For this review, take the finished solid that the model builds, in its own axes (mm). A direction names the side the tool comes from. Round coordinates to 2 decimals unless told otherwise and drop trailing zeros. Loops run counter-clockwise (first coordinate to the right, second up) from the corner with the lowest first, then second, coordinate; pieces in that order, holes last. Notation, with made-up numbers: M 31.5,-8 L 90.5,-8 A30 ccw 90.5,16 Z; hole C 62,82.25 d7. An arc over 180 degrees is marked long. Write item = value, one per line. Start each with the question number.
Autodesk Inventor part; units mm, degrees
ref_plane "YZ Plane" through (0, 0, 0) normal (1, 0, 0) x (0, 1, 0)
ref_plane "XZ Plane" through (0, 0, 0) normal (0, 1, 0) x (-1, 0, 0)
ref_plane "XY Plane" through (0, 0, 0) normal (0, 0, 1) x (1, 0, 0)
sketch "Sketch2" plane through (0, 0, 0) normal (1, 0, 0) x (0, 1, 0)
  line L0 (0, 0) -> (0, -17)
  line L1 (0, 0) -> (22, 0)
  line L2 (22, 0) -> (22, -15)
  line L3 (22, 0) -> (30, 0) construction
  line L4 (30, 0) -> (30, -17) construction
  line L5 (22, -17) -> (22, -15) construction
  line L6 (30, 0) -> (40, 0)
  line L7 (40, 0) -> (40, -34.5) construction
  line L8 (40, -34.5) -> (40, -32.5)
  line L9 (40, -32.5) -> (30, -15)
  line L10 (22, -15) -> (30, -15)
  line L11 (22, -15) -> (22, 0) construction
  line L12 (40, -34.5) -> (19.6496, -17)
  line L13 (19.6496, -17) -> (0, -17)
  dimension "d0" = 17
  dimension "d1" = 22
  dimension "d3" = 8
  dimension "d4" = 10
  dimension "d5" = 34.5
  dimension "d6" = 2
revolve "Revolution1" add sketch "Sketch2" angle 360 about axis through (0, 22, 0) along (0, 1, 0)
sketch "Sketch3" plane through (0, 22, 0) normal (0, 1, 0) x (1, 0, 0)
  line L0 (-3, -9.275) -> (3, -9.275)
  line L1 (3, -9.275) -> (3, 9.275)
  line L2 (3, 9.275) -> (-3, 9.275)
  line L3 (-3, 9.275) -> (-3, -9.275)
  line L4 (-3, -9.275) -> (3, 9.275) construction
  line L5 (3, -9.275) -> (-3, 9.275) construction
  point P0 (0, 0)
  dimension "d8" = 6
  dimension "d9" = 18.55
extrude "Extrusion1" cut sketch "Sketch3" against normal blind 15
sketch "Sketch4" plane through (0, 7, 0) normal (0, 1, 0) x (1, 0, 0)
  line L0 (-1.5, -8) -> (1.5, -8)
  line L1 (1.5, -8) -> (1.5, 8)
  line L2 (1.5, 8) -> (-1.5, 8)
  line L3 (-1.5, 8) -> (-1.5, -8)
  line L4 (-1.5, -8) -> (1.5, 8) construction
  line L5 (1.5, -8) -> (-1.5, 8) construction
  point P0 (0, 0)
  dimension "d12" = 3
  dimension "d13" = 16
extrude "Extrusion2" cut sketch "Sketch4" against normal blind 7
sketch "Sketch5" plane through (0, 0, 0) normal (0, -1, 0) x (1, 0, 0)
  line L0 (1.5, -8) -> (1.5, 8)
  line L1 (1.5, -8) -> (17.518, -8)
  line L2 (17.518, -8) -> (17.518, 8)
  line L3 (17.518, 8) -> (1.5, 8)
  line L4 (1.5, 8) -> (1.5, -8)
  point P0 (0, 0)
extrude "Extrusion3" cut sketch "Sketch5" against normal blind 4
properties part number "fitted nu funnel easy angle"
(1) For pin 1 Ø4.5 at (x, z) = (9, -0.5) entering from -Y; pin 2 Ø5 at (x, z) = (12.5, -20.5) entering from -Y; pin 3 Ø16.5 at (y, z) = (14.5, 0.5) entering from -X; pin 4 Ø1 at (x, z) = (-1.5, -10.5) entering from -Y, all flat-tipped, find the tip position at first contact; note any pin that passes through.
(2) Draft analysis for pull direction Z (two halves, no side actions). For faces 6 (the flat face through (3, 15, 0)), 7 (the flat face through (31, 40, -13)), 8 (the cylindrical face through (-16.596, 9.687, 3.685)), state which applies: +Z half, -Z half, draft (parallel to the pull), parting line (faces both ways), or undercut.
(3) Add section D-D on y = 31. Write out the cut boundary in (x, z), and give its area (3 significant figures).
(4) Add section A-A on z = 0. Write out the cut boundary in (x, y), and give its area (3 significant figures).
(5) Wall thickness on L1, parallel to Y at x = 6.5, z = -8.5; L2, parallel to Z at x = 0, y = 27.25; L3, parallel to Z at x = 0, y = 28.25: over which ranges is each line inside the solid? List them lowest first.
(6) Add section B-B on x = 0. Write out the cut boundary in (y, z) (3 decimals), and give its area (3 significant figures).
(7) Tool access review of faces 1 (the flat face through (5, 3, 8)), 2 (the flat face through (-5, 0, 0)), 3 (the flat face through (-1.5, 4, 0)), 4 (the flat face through (9, 4, 0)), 5 (the flat face through (-3, 15, 0)): name each direction out of +Z, -Z, +X, -X, +Y, -Y from which nothing blocks a thin tool from reaching the whole face with its end or side.
(8) Add section C-C on y = 11.5. Write out the cut boundary in (x, z) (3 decimals).
Answer sheet:
q1.pin_1 = 4
q1.pin_2 = 24.89
q1.pin_3 = -19.66
q1.pin_4 = 0
q2.face_6 = undercut
q2.face_7 = draft
q2.face_8 = parting line
q3.outline = C 0,0 d53.52; hole C 0,0 d33.5
q3.area = 1,370 mm²
q4.outline = M -34.5,40 L -17,19.65 L -17,0 L -1.5,0 L -1.5,7 L -3,7 L -3,22 L -15,22 L -15,30 L -32.5,40 Z; M 1.5,4 L 17,4 L 17,19.65 L 34.5,40 L 32.5,40 L 15,30 L 15,22 L 3,22 L 3,7 L 1.5,7 Z
q4.area = 828 mm²
q5.L1 = 0 to 22
q5.L2 = -23.54 to -15, 15 to 23.54
q5.L3 = -24.4 to -15, 15 to 24.4
q6.outline = M 0,-17 L 19.65,-17 L 40,-34.5 L 40,-32.5 L 30,-15 L 22,-15 L 22,-9.275 L 7,-9.275 L 7,-8 L 0,-8 Z; M 0,8 L 7,8 L 7,9.275 L 22,9.275 L 22,15 L 30,15 L 40,32.5 L 40,34.5 L 19.65,17 L 0,17 Z
q6.area = 611 mm²
q7.face_1 = -Y
q7.face_2 = +Z, -Z, +X, -X, -Y
q7.face_3 = +Y, -Y
q7.face_4 = +X, -Y
q7.face_5 = +Y
q8.outline = C 0,0 d34; hole M -3,-9.275 L 3,-9.275 L 3,9.275 L -3,9.275 Z
